Part model, mm, in its own coordinate system. Face numbers are marked on the shaded views. A direction names the side the tool comes from. Give positions to 0.01 mm unless a question says otherwise; leave off trailing zeros. Order: outer loops, then holes, each group sorted by start corner. A loop starts at its lowest first (then second) coordinate and runs counter-clockwise, first axis right, second up. Notation, with made-up numbers: M 81,48 L 107,48 A15 cw 107,64 Z; hole C -23.75,-10 d8. An arc over 180 degrees is marked long. Write each question's results on one line, items separated by ' | '. Start each with the question number.
from build123d import *

# Parameters (mm, degrees)
F1_DEPTH      = 90
F3_DEPTH      = 34.6420161514
F3_DEPTH_BACK = 34.6420161514


with BuildPart() as f1:
    # F0 (on Top) → F1 (new body)
    with BuildSketch(Plane.XY):
        Polygon((-20, 34.6410161514), (-40, 0), (-20, -34.6410161514), (20, -34.6410161514), (40, 0), (20, 34.6410161514), align=None)
    extrude(amount=F1_DEPTH)

    # F2 (on Front) → F3 (cut, two sides)
    with BuildSketch(Plane.XZ) as f3_sk:
        Polygon((-43.1388012565, 92.6622778185), (-43.1388012565, 20), (25, 20), (25, 40), (-30, 70), (-30, 92.6622778185), align=None)
    extrude(amount=-F3_DEPTH, mode=Mode.SUBTRACT)
    extrude(f3_sk.sketch, amount=F3_DEPTH_BACK, mode=Mode.SUBTRACT)


solid = f1.part
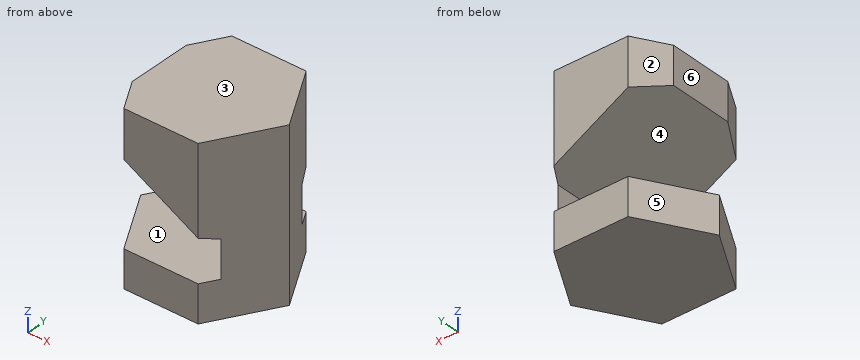
(1) Pull direction Z, two halves, no side cores. Call the marked faces 1, 2, 3 and 4: +Z half, -Z half, draft (parallel to the pull), parting line (faces both ways), or undercut.
(2) Probe L1, parallel to Z at x = -7, y = 29.5; L2, parallel to Y at x = 25, z = 66; L3, parallel to Z at x = -19, y = -20.5. List the from-to ranges inside material, lowest first.
(3) Tool access for the marked faces 5 and 6: list every direction of +Z, -Z, +X, -X, +Y, -Y with a clear straight run to the whole face (end or side of a thin tool).
(4) Saw through at D-D on y = 22. Give the cut face in (x, z), plus the area to 3 significant figures.
(5) Saw through at A-A on x = -22.5. Give the cut face in (y, z), plus the area to 3 significant figures.
(6) Drop flat-ended pins along their axis: P1, Ø1, axis at y = -12.5, z = 42.5, coming from the -X side; P2, Ø1.5, axis at y = -7.5, z = 48.5, coming from the +X side; P3, Ø6, axis at y = -7, z = 33, coming from the -X side. Give the stop position or say it passes through.
(7) Saw through at B-B on y = 30. Give the cut face in (x, z).
(8) Saw through at C-C on z = 6.5. Give the cut face in (x, y).
Taken from the geometry:
1) face 1: undercut | face 2: draft | face 3: +Z half | face 4: undercut
2) L1: z = 0 to 20, 57.45 to 90 | L2: y = -25.98 to 25.98 | L3: z = 0 to 20, 64 to 90
3) face 5: +Z, -Z, -X, +Y | face 6: +Z, -X, +Y, -Y
4) outline: M -27.3,0 L 27.3,0 L 27.3,90 L -27.3,90 L -27.3,68.53 L 25,40 L 25,20 L -27.3,20 Z | area: 3,120 mm²
5) outline: M -30.31,0 L 30.31,0 L 30.31,20 L -30.31,20 Z; M -30.31,65.91 L 30.31,65.91 L 30.31,90 L -30.31,90 Z | area: 2,670 mm²
6) P1: stops at x = 19.5 | P2: stops at x = 36.1 | P3: stops at x = 25
7) outline: M -22.68,0 L 22.68,0 L 22.68,20 L -22.68,20 Z; M -22.68,66.01 L 22.68,41.27 L 22.68,90 L -22.68,90 Z
8) outline: M -40,0 L -20,-34.64 L 20,-34.64 L 40,0 L 20,34.64 L -20,34.64 Z
